from build123d import *

# Parameters (mm, degrees)
BOSS_EXTRUDE1_DEPTH = 125
CUT_EXTRUDE1_DEPTH  = 17
SKETCH3_W           = 95
SKETCH3_H           = 69.22757419
CUT_EXTRUDE2_DEPTH  = 34
SKETCH4_W           = 25
SKETCH4_H           = 13.27242581
BOSS_EXTRUDE2_DEPTH = 3
SKETCH5_R           = 4
CUT_EXTRUDE3_DEPTH  = 26
SKETCH6_R           = 37.5
CUT_EXTRUDE4_DEPTH  = 3
BOSS_EXTRUDE3_DEPTH = 3
BOSS_EXTRUDE4_DEPTH = 3
BOSS_EXTRUDE5_DEPTH = 3


with BuildPart() as part:
    # Sketch1 → Boss-Extrude1 (new body)
    with BuildSketch(Plane(origin=(0, 0, 0), x_dir=(0, 0, -1), z_dir=(1, 0, 0))):
        Polygon((0, 0), (-220, 0), (-220, 45), (-121.223885949, 74.203491429), (9.810612088, 54.551256842), align=None)
        Polygon((-177.49762675, 52.35202023), (-120.869266543, 69.094386012), (-93.423815393, 64.978184153), (-93.423815393, 54.551256842), align=None, mode=Mode.SUBTRACT)
    extrude(amount=-BOSS_EXTRUDE1_DEPTH)

    # Sketch2 → Cut-Extrude1 (cut)
    with BuildSketch(Plane(origin=(0, 101.19793775, 29.919511777), x_dir=(1, 0, 0), z_dir=(0, 0.9589658804644564, 0.28352149848826236))):
        Polygon((-110, -159.280040992), (-15, -159.280040992), (-5, -149.280040992), (-5, -110.211285439), (-15, -100.211285439), (-110, -100.211285439), (-120, -110.211285439), (-120, -149.280040992), align=None)
    extrude(amount=-CUT_EXTRUDE1_DEPTH, mode=Mode.SUBTRACT)

    # Sketch3 → Cut-Extrude2 (cut)
    with BuildSketch(Plane(origin=(0, 54.790217418, -8.217303244), x_dir=(1, 0, 0), z_dir=(0, 0.9889396078246219, -0.1483187515983168))):
        with Locations((-62.5, -48.002658537)):
            Rectangle(SKETCH3_W, SKETCH3_H)
    extrude(amount=-CUT_EXTRUDE2_DEPTH, mode=Mode.SUBTRACT)

    # Sketch4 → Boss-Extrude2 (add)
    with BuildSketch(Plane(origin=(0, 54.790217418, -8.217303244), x_dir=(1, 0, 0), z_dir=(0, 0.9889396078246219, -0.1483187515983168))):
        with Locations((-62.5, -109.252658537)):
            Rectangle(SKETCH4_W, SKETCH4_H)
    extrude(amount=BOSS_EXTRUDE2_DEPTH)

    # Sketch5 → Cut-Extrude3 (cut)
    with BuildSketch(Plane(origin=(0, 57.757036242, -8.662259499), x_dir=(1, 0, 0), z_dir=(0, 0.988939607824622, -0.1483187515983164))):
        with Locations(Location((-62.5, -109.252658537, 0), (0, 0, 270))):
            Circle(SKETCH5_R)
    extrude(amount=-CUT_EXTRUDE3_DEPTH, mode=Mode.SUBTRACT)

    # Sketch6 → Cut-Extrude4 (cut)
    with BuildSketch(Plane(origin=(0, 0, 0), x_dir=(0, 0, -1), z_dir=(1, 0, 0))):
        with Locations((-182, -15)):
            Circle(SKETCH6_R)
        with Locations((-40, -15)):
            Circle(SKETCH6_R)
    cut_extrude4 = extrude(amount=-CUT_EXTRUDE4_DEPTH, mode=Mode.SUBTRACT)

    # Mirror1: Cut-Extrude4 across plane
    add(cut_extrude4.mirror(Plane(origin=(-62.5, 0, 0), x_dir=(0, 0, 1), z_dir=(1, 0, 0))), mode=Mode.SUBTRACT)

    # Sketch7 → Boss-Extrude3 (add)
    with BuildSketch(Plane.XY.offset(220)):
        Polygon((-113, 12), (-125, 12), (-125, 0), (0, 0), (0, 12), (-12, 12), align=None)
    extrude(amount=BOSS_EXTRUDE3_DEPTH)

    # Sketch8 → Boss-Extrude4 (add)
    with BuildSketch(Plane(origin=(0, 0, 0), x_dir=(0, 0, -1), z_dir=(1, 0, 0))):
        with BuildLine():
            Line((-81.487950058, 12), (-140.512049942, 12))
            ThreePointArc((-140.512049942, 12), (-171.177028416, 33.302311395), (-208, 27.121847063))
            ThreePointArc((-208, 27.121847063), (-214.976280656, 20.335654808), (-220, 12))
            Line((-220, 12), (-223, 12))
            Line((-223, 12), (-223, 0))
            Line((-223, 0), (-216.369317712, 0))
            ThreePointArc((-216.369317712, 0), (-182, 22.5), (-147.630682288, 0))
            Line((-147.630682288, 0), (-74.369317712, 0))
            ThreePointArc((-74.369317712, 0), (-40, 22.5), (-5.630682288, 0))
            Line((-5.630682288, 0), (0, 0))
            Line((0, 0), (1.221081194, 6.789740871))
            ThreePointArc((1.221081194, 6.789740871), (-2.437755356, 15.390427261), (-8.085309053, 22.837844835))
            ThreePointArc((-8.085309053, 22.837844835), (-47.230251909, 33.969107173), (-81.487950058, 12))
        make_face()
    boss_extrude4 = extrude(amount=BOSS_EXTRUDE4_DEPTH)

    # Mirror2: Boss-Extrude4 across plane
    add(boss_extrude4.mirror(Plane(origin=(-62.5, 0, 0), x_dir=(0, 0, 1), z_dir=(1, 0, 0))))

    # Sketch9 → Boss-Extrude5 (add)
    with BuildSketch(Plane(origin=(0, 0, 0), x_dir=(-1, 0, 0), z_dir=(0, -0.17700245783771668, -0.9842104093736296))):
        Polygon((12, 12), (0, 12), (0, 6.898668015), (-3, 6.898668015), (-3, 0), (128, 0), (128, 6.898668015), (125, 6.898668015), (125, 12), (113, 12), align=None)
    extrude(amount=BOSS_EXTRUDE5_DEPTH)


solid = part.part
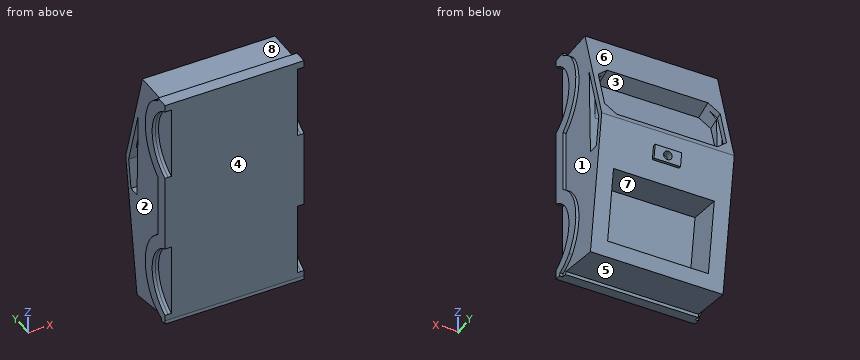
Geometry: final body of the model. Coordinates: model frame, mm. Face numbers are marked on the shaded views. A direction names the side the tool comes from. Round coordinates to 2 decimals unless told otherwise and drop trailing zeros. Loops run counter-clockwise (first coordinate to the right, second up) from the corner with the lowest first, then second, coordinate; pieces in that order, holes last. Notation, with made-up numbers: M 81,67.5 L 92,67.5 A4 cw 92,71.5 Z; hole C 71,34.25 d8. An arc over 180 degrees is marked long. Put each result on its own line as item: value. Start each with the question number.
(1) Set-up query: the marked faces 1, 2, 3 and 4. Return all of +Z, -Z, +X, -X, +Y, -Y with unobstructed straight access to the full face (end or side cutting, diameter ignored); none if empty.
(2) Section query D-D (z = 19). Return loops of the section in (x, y), then the cut area to 3 significant figures.
(3) Section query A-A (x = -27.5). Return loops of the section in (y, z), then the cut area to 3 significant figures.
(4) Contact query for flat-ended pins moving along their axis: pin 1 Ø7 at (y, z) = (8.5, 24) entering from -X; pin 2 Ø25 at (y, z) = (10.5, 173) entering from +X; pin 3 Ø20.5 at (y, z) = (47, 84) entering from -X; pin 4 Ø1.5 at (x, z) = (-88.5, 221.5) entering from +Y. Output: stop coordinate, or through.
(5) Material intervals for line 1 along X through (y, z) = (58, 169.5); line 2 along X through (y, z) = (61.5, 49); line 3 along X through (y, z) = (3, 31), sorted ascending. Write a range as [from, to].
(6) Draft query along Y for the marked faces 5, 6, 7 and 8. Return one class per face: +Y half, -Y half, draft (parallel to the pull), parting line (faces both ways), or undercut.
(7) Section query C-C (z = 58). Return loops of the section in (x, y).
(8) Section query B-B (z = 165). Return loops of the section in (x, y).
Findings below:
1. face 1: +X, +Y
1. face 2: -X, +Y
1. face 3: +Y
1. face 4: +Z, +X, -X, -Y
2. outline: M -128,16.07 L -122,16.07 L -122,0 L -3,0 L -3,16.07 L 3,16.07 L 3,29.82 L 0,29.82 L 0,58.87 L -15,58.87 L -15,24.49 L -110,24.49 L -110,58.87 L -125,58.87 L -125,29.82 L -128,29.82 Z
2. area: 4,080 mm2
3. outline: M -0.53,-2.95 L 11.28,-5.08 L 11.81,-2.12 L 54.55,-9.81 L 56.78,5.02 L 23.15,10.07 L 33.42,78.53 L 67.04,73.49 L 74.2,121.22 L 72.79,126.02 L 67.99,124.6 L 69.09,120.87 L 64.98,93.42 L 54.55,93.42 L 53.57,131.06 L 39.74,177.84 L 56.04,182.66 L 45,220 L 12,220 L 12,223 L 0,223 L 0,0 Z
3. area: 10,400 mm2
4. pin 1: stops at x = -122
4. pin 2: stops at x = 3
4. pin 3: stops at x = -125
4. pin 4: stops at y = 12
5. line 1: x = [-125, -120], [-5, 0]
5. line 2: x = [-125, -110], [-15, 0]
5. line 3: x = [-122, -3]
6. face 5: undercut
6. face 6: +Y half
6. face 7: undercut
6. face 8: draft
7. outline: M -128,17.9 L -122,17.9 L -122,0 L -3,0 L -3,17.9 L 3,17.9 L 3,31.11 L 0,31.11 L 0,64.72 L -15,64.72 L -15,30.34 L -110,30.34 L -110,64.72 L -125,64.72 L -125,31.11 L -128,31.11 Z
8. outline: M -128,18.43 L -122,18.43 L -122,0 L -3,0 L -3,18.43 L 3,18.43 L 3,31.49 L 0,31.49 L 0,52.68 L -5,52.68 L -5,43.53 L -120,43.53 L -120,52.68 L -125,52.68 L -125,31.49 L -128,31.49 Z; M -125,56.05 L -120,56.05 L -120,61.26 L -125,61.26 Z; M -5,56.05 L 0,56.05 L 0,61.26 L -5,61.26 Z
